from build123d import *

# Parameters (mm, degrees)
SKETCH1_R           = 12.7
BOSS_EXTRUDE1_DEPTH = 2.54
SKETCH2_R           = 10.172184257
BOSS_EXTRUDE2_DEPTH = 2.54
FILLET1_R           = 0.762
FILLET2_R           = 0.762


with BuildPart() as part:
    # Sketch1 → Boss-Extrude1 (new body)
    with BuildSketch(Plane(origin=(0, 0, 0), x_dir=(1, 0, 0), z_dir=(0, 1, 0))):
        with Locations(Location((0, 0, 0), (0, 0, 270))):
            Circle(SKETCH1_R)
    extrude(amount=BOSS_EXTRUDE1_DEPTH)

    # Sketch2 → Boss-Extrude2 (add)
    with BuildSketch(Plane(origin=(0, 2.54, 0), x_dir=(1, 0, 0), z_dir=(0, 1, 0))):
        with Locations(Location((0, 0, 0), (0, 0, 270))):
            Circle(SKETCH2_R)
    extrude(amount=BOSS_EXTRUDE2_DEPTH)

    # Fillet1
    fillet1_edges = [part.edges().sort_by_distance(p)[0] for p in [
        (0, 2.54, -12.7),
    ]]
    fillet(fillet1_edges, radius=FILLET1_R)

    # Fillet2
    fillet2_edges = [part.edges().sort_by_distance(p)[0] for p in [
        (0, 5.08, -10.172184257),
    ]]
    fillet(fillet2_edges, radius=FILLET2_R)


solid = part.part
Design review of the part built by this model. Coordinates are the model's own, in mm. A direction names the side the tool comes from. Coordinates: 2 decimals unless noted, no trailing zeros. Loops run counter-clockwise (first coordinate to the right, second up) from the corner with the lowest first, then second, coordinate; pieces in that order, holes last. Notation, with made-up numbers: (33.25, -33.5) -> (76.25, -33.5) arc R26 cw to (76.25, 2.5) -> close; hole circle Ø7 at (35, 20.25). An arc over 180 degrees is marked (long way). Use a Markdown table: item, result. Add a question column.
Item 1: We need section C-C, the plane y = 1.3. Write out the cut boundary in (x, z).
Item 2: Wall thickness on L1, parallel to Y at x = 1, z = -11; L2, parallel to X at y = 2.15, z = 11; L3, parallel to X at y = 4.7, z = 6.75: over which ranges is each line inside the solid? List them lowest first. Write a range as from..to.
Item 3: We need section B-B, the plane z = 0. Write out the cut boundary in (x, y), and give its area (3 significant figures).
Item 4: Machinability: for faces 1 (the cylindrical face through (-6.19, 3.42, -8.07)), 2 (the flat face through (0, 0, 0)), which of the approach directions +Z, -Z, +X, -X, +Y, -Y give a long, thin tool a straight path to every point of the face, cutting with its end or side? Answer none if there is none.
Item 5: We need section A-A, the plane x = 0. Write out the cut boundary in (y, z).
Item 6: Clearance check with flat-ended pins moving along their axes: P1, Ø10, axis at x = 1.5, z = 1, coming from the -Y side; P2, Ø1.5, axis at x = 4, y = 1, coming from the -Z side. State where each tip first meets the part, or that it passes through.
Numbers:
| question | item | result |
|---|---|---|
| 1 | outline | circle Ø25.4 at (0, 0) |
| 2 | L1 | y = 0..2.54 |
| 2 | L2 | x = -6.15..6.15 |
| 2 | L3 | x = -7.47..7.47 |
| 3 | outline | (-12.7, 0) -> (12.7, 0) -> (12.7, 1.78) arc R0.76 ccw to (11.94, 2.54) -> (10.17, 2.54) -> (10.17, 4.32) arc R0.76 ccw to (9.41, 5.08) -> (-9.41, 5.08) arc R0.76 ccw to (-10.17, 4.32) -> (-10.17, 2.54) -> (-11.94, 2.54) arc R0.76 ccw to (-12.7, 1.78) -> close |
| 3 | area | 116 mm^2 |
| 4 | face 1 | +Y |
| 4 | face 2 | +Z, -Z, +X, -X, -Y |
| 5 | outline | (0, -12.7) -> (1.78, -12.7) arc R0.76 ccw to (2.54, -11.94) -> (2.54, -10.17) -> (4.32, -10.17) arc R0.76 ccw to (5.08, -9.41) -> (5.08, 9.41) arc R0.76 ccw to (4.32, 10.17) -> (2.54, 10.17) -> (2.54, 11.94) arc R0.76 ccw to (1.78, 12.7) -> (0, 12.7) -> close |
| 6 | P1 | stops at y = 0 |
| 6 | P2 | stops at z = -12.28 |
